Autodesk Inventor part; units mm, degrees
ref_plane "YZ Plane" through (0, 0, 0) normal (1, 0, 0) x (0, 1, 0)
ref_plane "XZ Plane" through (0, 0, 0) normal (0, 1, 0) x (-1, 0, 0)
ref_plane "XY Plane" through (0, 0, 0) normal (0, 0, 1) x (1, 0, 0)
sketch "Sketch1" plane through (0, 0, 0) normal (1, 0, 0) x (0, 1, 0)
  line L0 (-15.875, 38.1) -> (15.875, 38.1)
  line L1 (25.4, 28.575) -> (25.4, -28.575)
  line L2 (15.875, -38.1) -> (-15.875, -38.1)
  line L3 (-25.4, -28.575) -> (-25.4, 28.575)
  line L4 (-25.4, 38.1) -> (25.4, -38.1) construction
  line L5 (25.4, 38.1) -> (-25.4, -38.1) construction
  arc A0 (25.4, 28.575) -> (15.875, 38.1) centre (15.875, 28.575) ccw
  arc A1 (-15.875, 38.1) -> (-25.4, 28.575) centre (-15.875, 28.575) ccw
  arc A2 (-25.4, -28.575) -> (-15.875, -38.1) centre (-15.875, -28.575) ccw
  arc A3 (15.875, -38.1) -> (25.4, -28.575) centre (15.875, -28.575) ccw
  line L6 (22.225, -28.575) -> (22.225, 28.575)
  arc A4 (22.225, 28.575) -> (15.875, 34.925) centre (15.875, 28.575) ccw
  line L7 (15.875, 34.925) -> (-15.875, 34.925)
  arc A5 (-15.875, 34.925) -> (-22.225, 28.575) centre (-15.875, 28.575) ccw
  line L8 (-22.225, 28.575) -> (-22.225, -28.575)
  arc A6 (-22.225, -28.575) -> (-15.875, -34.925) centre (-15.875, -28.575) ccw
  line L9 (-15.875, -34.925) -> (15.875, -34.925)
  arc A7 (15.875, -34.925) -> (22.225, -28.575) centre (15.875, -28.575) ccw
  point P0 (0, 0)
  dimension "d0" = 50.8
  dimension "d1" = 76.2
  dimension "d2" = 9.525
  dimension "d3" = 3.175
extrude "Extrusion1" add sketch "Sketch1" along normal blind 1060.45
equation "\"d0\" = stockHeight"
equation "\"d1\" = stockWidth"
equation "\"d2\" = stockRad"
equation "\"d3\" = stockGuage"
equation "\"d4\" = baseWidth - 2 * capThickness"
equation "\"height\" = 203.2"
equation "\"shaftDiam\" = 6.35"
equation "\"shaftSpace\" = 1.5875"
equation "\"stageSpace\" = 2.54"
equation "\"stageAngle\" = 15deg"
equation "\"stockHeight\" = 50.8"
equation "\"stockWidth\" = 76.2"
equation "\"stockRad\" = 9.525"
equation "\"stockGuage\" = 3.175"
equation "\"groundActu\" = 304.8"
equation "\"baseWidth\" = 1066.8"
equation "\"baseDepth\" = 254"
equation "\"capThickness\" = 3.175"
equation "\"sup1Ang\" = 22.619865deg"
equation "\"sup1Len\" = 660.4"
equation "\"supVertLen\" = 955.13561"
equation "\"sup2Ang\" = 8.959949deg"
equation "\"sup2Len\" = 2079.37366"
equation "\"supSideAng\" = 19.376933deg"
equation "\"supSideLen\" = 1531.12879"
equation "\"FlangeDiam\" = 12.7"
equation "\"bearingDiam\" = 9.5504"
equation "\"FlangeDepth\" = 1.5875"
equation "\"smallFilet\" = 0.39687"
equation "\"thickness\" = 12.7"
equation "\"ringDiam\" = 96.46608"
properties part number "base bar" material "Aluminum 6061"
Can you work these out from the model? Positions are in its coordinate system, mm. A direction names the side the tool comes from. Coordinates: 2 decimals unless noted, no trailing zeros. Loops run counter-clockwise (first coordinate to the right, second up) from the corner with the lowest first, then second, coordinate; pieces in that order, holes last.
1) Imagine slicing it at C-C on x = 747. List the corners of the cut face in (y, z) for me (3 decimals).
2) Thinking about a two-plate mould opening in Y: for faces 3 (the flat face through (523, -25.4, 0)), 4 (the flat face through (523, 22.225, 0)), 5 (the flat face through (0, -23, -5)), which applies, pulls with the +Y half, pulls with the -Y half, needs draft (parallel to the pull), parting line crosses it, or undercut?
3) Imagine slicing it at A-A on y = -6.5. List the corners of the cut face in (x, z) for me (3 decimals), plus the area to 3 significant figures.
4) For pin 1 (1.5 mm diameter, centred on x = 225.5, y = 20, fed in from +Z), with a flat end and sliding along its axis, tell me the tip position at first contact or that it passes through.
5) I need wall thicknesses on probe 1 along Z at (x, y) = (423.5, -13) (3 decimals); probe 2 along Y at (x, z) = (966.5, 17) (3 decimals); probe 3 along Y at (x, z) = (633.5, -33.5). Which ranges of each line are inside material? Lowest first, please.
6) Imagine slicing it at B-B on z = -15. List the corners of the cut face in (x, y) for me (3 decimals).
7) Which directions (+Z, -Z, +X, -X, +Y, -Y) give clear straight access to the entire face, cutting with the end or side of a thin tool? Please do faces 1 (the flat face through (523, 0, 38.1)), 2 (the flat face through (523, 0, -34.925)).
Completed:
1. outline: (-25.4, -28.575) arc R9.525 ccw to (-15.875, -38.1) - (15.875, -38.1) arc R9.525 ccw to (25.4, -28.575) - (25.4, 28.575) arc R9.525 ccw to (15.875, 38.1) - (-15.875, 38.1) arc R9.525 ccw to (-25.4, 28.575) - close; hole (-22.225, -28.575) arc R6.35 ccw to (-15.875, -34.925) - (15.875, -34.925) arc R6.35 ccw to (22.225, -28.575) - (22.225, 28.575) arc R6.35 ccw to (15.875, 34.925) - (-15.875, 34.925) arc R6.35 ccw to (-22.225, 28.575) - close
2. face 3: pulls with the -Y half
2. face 4: undercut
2. face 5: needs draft
3. outline: (0, -38.1) - (1060.45, -38.1) - (1060.45, -34.925) - (0, -34.925) - close; (0, 34.925) - (1060.45, 34.925) - (1060.45, 38.1) - (0, 38.1) - close
3. area: 6,730 mm2
4. pin 1: stops at z = 37.48
5. probe 1: z = -38.1 to -34.925, 34.925 to 38.1
5. probe 2: y = -25.4 to -22.225, 22.225 to 25.4
5. probe 3: y = -24.03 to -19.88, 19.88 to 24.03
6. outline: (0, -25.4) - (1060.45, -25.4) - (1060.45, -22.225) - (0, -22.225) - close; (0, 22.225) - (1060.45, 22.225) - (1060.45, 25.4) - (0, 25.4) - close
7. face 1: +Z, +X, -X, +Y, -Y
7. face 2: +X, -X
